Can you work these out from the model? Positions are in its coordinate system, mm. Face numbers are marked on the shaded views. A direction names the side the tool comes from. Coordinates: 2 decimals unless noted, no trailing zeros. Order: outer loops, then holes, each group sorted by start corner. A loop starts at its lowest first (then second) coordinate and runs counter-clockwise, first axis right, second up. Notation, with made-up numbers: (-12.5, -6) -> (23.5, -6) arc R24 ccw to (23.5, 6) -> close; hole circle Ø1 at (75, 13.25). An arc over 180 degrees is marked (long way). Answer in a Markdown table with one row per item.
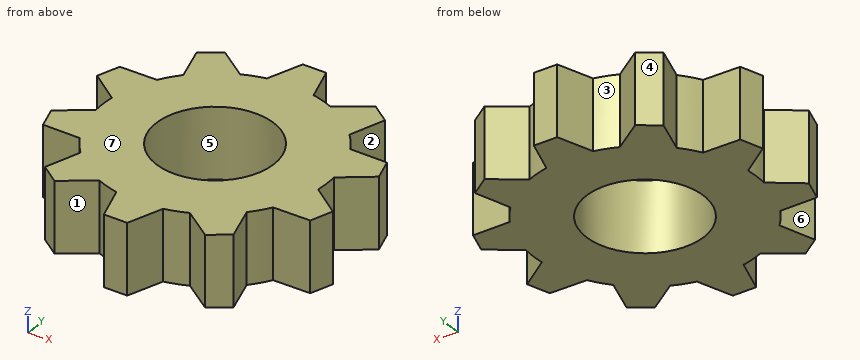
```python
from build123d import *

# Parameters (mm, degrees)
F0_R     = 4.7746482928
F0_R_2   = 2.5
F2_DEPTH = 3
F3_COUNT = 10
F3_ANGLE = 324


with BuildPart() as f2:
    # F0 (on Top) + F1 (on face) → F2 (new body)
    with BuildSketch(Plane.XY):
        Circle(F0_R)
        Circle(F0_R_2, mode=Mode.SUBTRACT)
    with BuildSketch(Plane.XY):
        with BuildLine():
            ThreePointArc((-1, 4.6687542578), (0, 4.7746482928), (1, 4.6687542578))
            Line((1, 4.6687542578), (0.5, 6.1687542578))
            Line((0.5, 6.1687542578), (-0.5, 6.1687542578))
            Line((-0.5, 6.1687542578), (-1, 4.6687542578))
        make_face()
    extrude(amount=F2_DEPTH)

    # F3: F2 ×10 about axis
    f3_axis = Axis((0, 0, 3), (0, 0, -1))


with BuildPart() as f2_1:
    add(f2.part)
    for i in range(1, F3_COUNT):
        add(f2.part.rotate(f3_axis, i * F3_ANGLE / (F3_COUNT - 1)))


solid = f2_1.part
```
(1) Will these pins go through, and if not, where does the flat tip stop? pin 1 Ø1.5 at (y, z) = (-4, 0.5) entering from +X; pin 2 Ø1.5 at (x, z) = (-4, 2) entering from +Y; pin 3 Ø1.5 at (x, z) = (4.5, 0.5) entering from +Y.
Response values:
| item | result |
|---|---|
| pin 1 | x = 4.03 |
| pin 2 | y = 5.26 |
| pin 3 | y = 4.9 |
(2) Suppose I cut it at B-B (x = 0). Please give me the cut outline in (y, z), and give its area (3 significant figures).
Response values:
| item | result |
|---|---|
| outline | (-6.17, 0) -> (-2.5, 0) -> (-2.5, 3) -> (-6.17, 3) -> close; (2.5, 0) -> (6.17, 0) -> (6.17, 3) -> (2.5, 3) -> close |
| area | 22.0 mm2 |
(3) I need wall thicknesses on line 1 (X direction, y = 0, z = 0.75); line 2 (Y direction, x = 0, z = 1.8); line 3 (X direction, y = 5, z = 2.05). Which ranges of each line are inside material? Lowest first, please. Write a range as [from, to].
Response values:
| item | result |
|---|---|
| line 1 | [-4.77, -2.5], [2.5, 4.77] |
| line 2 | [-6.17, -2.5], [2.5, 6.17] |
| line 3 | [-3.61, -2.82], [-0.89, 0.89], [2.82, 3.61] |
(4) Suppose I cut it at A-A (y = 0). Please give me the cut outline in (x, z).
Response values:
| item | result |
|---|---|
| outline | (-4.77, 0) -> (-2.5, 0) -> (-2.5, 3) -> (-4.77, 3) -> close; (2.5, 0) -> (4.77, 0) -> (4.77, 3) -> (2.5, 3) -> close |
(5) On a 3-axis mill with a long thin cutter (end or side, diameter ignored), from which of +Z, -Z, +X, -X, +Y, -Y can I reach the whole of each face in a straight line? I mean the marked faces 1, 2, 3 and 4. Say none if no direction works.
Response values:
| item | result |
|---|---|
| face 1 | +Z, -Z, -Y |
| face 2 | +Z, -Z, +X |
| face 3 | +Z, -Z, +Y |
| face 4 | +Z, -Z, -X, +Y |
(6) We'd pull the mould along X, two halves only. Please class the marked faces 5, 6 and 7: +X half, -X half, draft (parallel to the pull), parting line (faces both ways), or undercut.
Response values:
| item | result |
|---|---|
| face 5 | undercut |
| face 6 | -X half |
| face 7 | draft |
